Here's how the part is built. I have some questions about the finished solid (model axes, mm). A direction names the side the tool comes from. Round coordinates to 2 decimals unless told otherwise and drop trailing zeros. Order: outer loops, then holes, each group sorted by start corner. A loop starts at its lowest first (then second) coordinate and runs counter-clockwise, first axis right, second up.
```python
from build123d import *

# Parameters (mm, degrees)
SKETCH3_W           = 25.4
SKETCH3_H           = 25.4
BOSS_EXTRUDE1_DEPTH = 76.8
SKETCH4_R           = 2.6035
CUT_EXTRUDE1_DEPTH  = 79.872175068
CUT_EXTRUDE2_DEPTH  = 79.872175068
FILLET1_R           = 2.54
FILLET2_R           = 1.778


with BuildPart() as part:
    # Sketch3 → Boss-Extrude1 (new body)
    with BuildSketch(Plane.XY):
        Rectangle(SKETCH3_W, SKETCH3_H)
    extrude(amount=BOSS_EXTRUDE1_DEPTH)

    # Sketch4 → Cut-Extrude1 (cut, through all)
    with BuildSketch(Plane.XY.offset(76.8)):
        with BuildLine():
            Line((3.2512, 12.7), (-3.2512, 12.7))
            Line((-3.2512, 12.7), (-3.2512, 10.4902))
            Line((-3.2512, 10.4902), (-6.348478019, 10.4902))
            ThreePointArc((-6.348478019, 10.4902), (-7.335478831, 9.830707141), (-7.103895736, 8.666460301))
            Line((-7.103895736, 8.666460301), (-2.958635435, 4.5212))
            Line((-2.958635435, 4.5212), (2.958635435, 4.5212))
            Line((2.958635435, 4.5212), (7.103895736, 8.666460301))
            ThreePointArc((7.103895736, 8.666460301), (7.335478831, 9.830707141), (6.348478019, 10.4902))
            Line((6.348478019, 10.4902), (3.2512, 10.4902))
            Line((3.2512, 10.4902), (3.2512, 12.7))
        make_face()
        with BuildLine():
            Line((12.7, -3.2512), (12.7, 3.2512))
            Line((12.7, 3.2512), (10.4902, 3.2512))
            Line((10.4902, 3.2512), (10.4902, 6.348478019))
            ThreePointArc((10.4902, 6.348478019), (9.830707141, 7.335478831), (8.666460301, 7.103895736))
            Line((8.666460301, 7.103895736), (4.5212, 2.958635435))
            Line((4.5212, 2.958635435), (4.5212, -2.958635435))
            Line((4.5212, -2.958635435), (8.666460301, -7.103895736))
            ThreePointArc((8.666460301, -7.103895736), (9.830707141, -7.335478831), (10.4902, -6.348478019))
            Line((10.4902, -6.348478019), (10.4902, -3.2512))
            Line((10.4902, -3.2512), (12.7, -3.2512))
        make_face()
        with BuildLine():
            Line((-3.2512, -10.4902), (-3.2512, -12.7))
            Line((-3.2512, -12.7), (3.2512, -12.7))
            Line((3.2512, -12.7), (3.2512, -10.4902))
            Line((3.2512, -10.4902), (6.348478019, -10.4902))
            ThreePointArc((6.348478019, -10.4902), (7.335478831, -9.830707141), (7.103895736, -8.666460301))
            Line((7.103895736, -8.666460301), (2.958635435, -4.5212))
            Line((2.958635435, -4.5212), (-2.958635435, -4.5212))
            Line((-2.958635435, -4.5212), (-7.103895736, -8.666460301))
            ThreePointArc((-7.103895736, -8.666460301), (-7.335478831, -9.830707141), (-6.348478019, -10.4902))
            Line((-6.348478019, -10.4902), (-3.2512, -10.4902))
        make_face()
        with BuildLine():
            Line((-10.4902, 3.2512), (-12.7, 3.2512))
            Line((-12.7, 3.2512), (-12.7, -3.2512))
            Line((-12.7, -3.2512), (-10.4902, -3.2512))
            Line((-10.4902, -3.2512), (-10.4902, -6.348478019))
            ThreePointArc((-10.4902, -6.348478019), (-9.830707141, -7.335478831), (-8.666460301, -7.103895736))
            Line((-8.666460301, -7.103895736), (-4.5212, -2.958635435))
            Line((-4.5212, -2.958635435), (-4.5212, 2.958635435))
            Line((-4.5212, 2.958635435), (-8.666460301, 7.103895736))
            ThreePointArc((-8.666460301, 7.103895736), (-9.830707141, 7.335478831), (-10.4902, 6.348478019))
            Line((-10.4902, 6.348478019), (-10.4902, 3.2512))
        make_face()
        Circle(SKETCH4_R)
    extrude(amount=-CUT_EXTRUDE1_DEPTH, mode=Mode.SUBTRACT)

    # Sketch5 → Cut-Extrude2 (cut, through all)
    with BuildSketch(Plane.XY.offset(76.8)):
        with BuildLine():
            ThreePointArc((-11.5951, 3.2512), (-12.376382283, 3.574817717), (-12.7, 4.3561))
            Line((-12.7, 4.3561), (-12.7, 3.2512))
            Line((-12.7, 3.2512), (-11.5951, 3.2512))
        make_face()
        with BuildLine():
            ThreePointArc((-10.4902, 4.3561), (-10.813817717, 3.574817717), (-11.5951, 3.2512))
            Line((-11.5951, 3.2512), (-10.4902, 3.2512))
            Line((-10.4902, 3.2512), (-10.4902, 4.3561))
        make_face()
        with BuildLine():
            Line((-12.7, -3.2512), (-12.7, -4.3561))
            ThreePointArc((-12.7, -4.3561), (-12.376382283, -3.574817717), (-11.5951, -3.2512))
            Line((-11.5951, -3.2512), (-12.7, -3.2512))
        make_face()
        with BuildLine():
            Line((-10.4902, -3.2512), (-11.5951, -3.2512))
            ThreePointArc((-11.5951, -3.2512), (-10.813817717, -3.574817717), (-10.4902, -4.3561))
            Line((-10.4902, -4.3561), (-10.4902, -3.2512))
        make_face()
        with BuildLine():
            Line((-3.2512, -11.595100007), (-3.2512, -10.4902))
            Line((-3.2512, -10.4902), (-4.3561, -10.4902))
            ThreePointArc((-4.3561, -10.4902), (-3.574817715, -10.81381772), (-3.2512, -11.595100007))
        make_face()
        with BuildLine():
            Line((-3.2512, -12.7), (-3.2512, -11.595100007))
            ThreePointArc((-3.2512, -11.595100007), (-3.57481772, -12.376382285), (-4.3561, -12.7))
            Line((-4.3561, -12.7), (-3.2512, -12.7))
        make_face()
        with BuildLine():
            Line((3.2512, -10.4902), (3.2512, -11.5951))
            ThreePointArc((3.2512, -11.5951), (3.574817718, -10.813817717), (4.3561, -10.4902))
            Line((4.3561, -10.4902), (3.2512, -10.4902))
        make_face()
        with BuildLine():
            Line((3.2512, -12.7), (4.3561, -12.7))
            ThreePointArc((4.3561, -12.7), (3.574817717, -12.376382282), (3.2512, -11.5951))
            Line((3.2512, -11.5951), (3.2512, -12.7))
        make_face()
        with BuildLine():
            Line((11.5951, -3.2512), (10.4902, -3.2512))
            Line((10.4902, -3.2512), (10.4902, -4.3561))
            ThreePointArc((10.4902, -4.3561), (10.813817717, -3.574817717), (11.5951, -3.2512))
        make_face()
        with BuildLine():
            Line((12.7, -3.2512), (11.5951, -3.2512))
            ThreePointArc((11.5951, -3.2512), (12.376382283, -3.574817717), (12.7, -4.3561))
            Line((12.7, -4.3561), (12.7, -3.2512))
        make_face()
        with BuildLine():
            Line((10.4902, 3.2512), (11.5951, 3.2512))
            ThreePointArc((11.5951, 3.2512), (10.813817717, 3.574817717), (10.4902, 4.3561))
            Line((10.4902, 4.3561), (10.4902, 3.2512))
        make_face()
        with BuildLine():
            Line((12.7, 3.2512), (12.7, 4.3561))
            ThreePointArc((12.7, 4.3561), (12.376382283, 3.574817717), (11.5951, 3.2512))
            Line((11.5951, 3.2512), (12.7, 3.2512))
        make_face()
        with BuildLine():
            Line((3.2512, 12.7), (3.2512, 11.595099996))
            ThreePointArc((3.2512, 11.595099996), (3.574817716, 12.376382281), (4.3561, 12.7))
            Line((4.3561, 12.7), (3.2512, 12.7))
        make_face()
        with BuildLine():
            Line((3.2512, 11.595099996), (3.2512, 10.4902))
            Line((3.2512, 10.4902), (4.3561, 10.4902))
            ThreePointArc((4.3561, 10.4902), (3.574817719, 10.813817716), (3.2512, 11.595099996))
        make_face()
        with BuildLine():
            Line((-3.2512, 12.7), (-4.3561, 12.7))
            ThreePointArc((-4.3561, 12.7), (-3.574817717, 12.376382283), (-3.2512, 11.5951))
            Line((-3.2512, 11.5951), (-3.2512, 12.7))
        make_face()
        with BuildLine():
            Line((-3.2512, 10.4902), (-3.2512, 11.5951))
            ThreePointArc((-3.2512, 11.5951), (-3.574817717, 10.813817717), (-4.3561, 10.4902))
            Line((-4.3561, 10.4902), (-3.2512, 10.4902))
        make_face()
        with BuildLine():
            ThreePointArc((-12.7, 5.23875), (-12.14755, 5.7912), (-12.7, 6.34365))
            Line((-12.7, 6.34365), (-12.7, 5.23875))
        make_face()
        with BuildLine():
            ThreePointArc((-12.7, 9.60755), (-12.14755, 10.16), (-12.7, 10.71245))
            Line((-12.7, 10.71245), (-12.7, 9.60755))
        make_face()
        with BuildLine():
            ThreePointArc((-10.71245, 12.7), (-10.16, 12.14755), (-9.60755, 12.7))
            Line((-9.60755, 12.7), (-10.71245, 12.7))
        make_face()
        with BuildLine():
            ThreePointArc((-6.34365, 12.7), (-5.7912, 12.14755), (-5.23875, 12.7))
            Line((-5.23875, 12.7), (-6.34365, 12.7))
        make_face()
        with BuildLine():
            Line((6.34365, 12.7), (5.23875, 12.7))
            ThreePointArc((5.23875, 12.7), (5.7912, 12.14755), (6.34365, 12.7))
        make_face()
        with BuildLine():
            Line((10.71245, 12.7), (9.60755, 12.7))
            ThreePointArc((9.60755, 12.7), (10.16, 12.14755), (10.71245, 12.7))
        make_face()
        with BuildLine():
            Line((12.7, 10.71245), (12.7, 9.60755))
            ThreePointArc((12.7, 9.60755), (12.14755, 10.16), (12.7, 10.71245))
        make_face()
        with BuildLine():
            Line((12.7, 6.34365), (12.7, 5.23875))
            ThreePointArc((12.7, 5.23875), (12.14755, 5.7912), (12.7, 6.34365))
        make_face()
        with BuildLine():
            Line((-12.7, -6.34365), (-12.7, -5.23875))
            ThreePointArc((-12.7, -5.23875), (-12.14755, -5.7912), (-12.7, -6.34365))
        make_face()
        with BuildLine():
            Line((-12.7, -10.71245), (-12.7, -9.60755))
            ThreePointArc((-12.7, -9.60755), (-12.14755, -10.16), (-12.7, -10.71245))
        make_face()
        with BuildLine():
            Line((-10.71245, -12.7), (-9.60755, -12.7))
            ThreePointArc((-9.60755, -12.7), (-10.16, -12.14755), (-10.71245, -12.7))
        make_face()
        with BuildLine():
            Line((-6.34365, -12.7), (-5.23875, -12.7))
            ThreePointArc((-5.23875, -12.7), (-5.7912, -12.14755), (-6.34365, -12.7))
        make_face()
        with BuildLine():
            Line((12.7, -10.71245), (12.7, -9.60755))
            ThreePointArc((12.7, -9.60755), (12.14755, -10.16), (12.7, -10.71245))
        make_face()
        with BuildLine():
            Line((12.7, -6.34365), (12.7, -5.23875))
            ThreePointArc((12.7, -5.23875), (12.14755, -5.7912), (12.7, -6.34365))
        make_face()
        with BuildLine():
            Line((10.71245, -12.7), (9.60755, -12.7))
            ThreePointArc((9.60755, -12.7), (10.16, -12.14755), (10.71245, -12.7))
        make_face()
        with BuildLine():
            Line((6.34365, -12.7), (5.23875, -12.7))
            ThreePointArc((5.23875, -12.7), (5.7912, -12.14755), (6.34365, -12.7))
        make_face()
    extrude(amount=-CUT_EXTRUDE2_DEPTH, mode=Mode.SUBTRACT)

    # Fillet1
    fillet1_edges = [part.edges().sort_by_distance(p)[0] for p in [
        (-2.958635435, -4.5212, 38.4),
        (2.958635435, -4.5212, 38.4),
        (4.5212, -2.958635435, 38.4),
        (4.5212, 2.958635435, 38.4),
        (-4.5212, 2.958635435, 38.4),
        (-4.5212, -2.958635435, 38.4),
        (2.958635435, 4.5212, 38.4),
        (-2.958635435, 4.5212, 38.4),
    ]]
    fillet(fillet1_edges, radius=FILLET1_R)

    # Fillet2
    fillet2_edges = [part.edges().sort_by_distance(p)[0] for p in [
        (-12.7, 12.7, 38.4),
        (12.7, 12.7, 38.4),
        (12.7, -12.7, 38.4),
        (-12.7, -12.7, 38.4),
    ]]
    fillet(fillet2_edges, radius=FILLET2_R)


solid = part.part
```
1) We'd pull the mould along X, two halves only. Please class faces 1 (the cylindrical face through (9.847, 7.329, 38.938)), 2 (the flat face through (12.7, -8, 38)), 3 (the flat face through (-8, 12.7, 38)): +X half, -X half, draft (parallel to the pull), parting line (faces both ways), or undercut.
2) I need wall thicknesses on line 1 (Y direction, x = 0, z = 58); line 2 (Y direction, x = -3.5, z = 69); line 3 (X direction, y = 5, z = 24.5). Which ranges of each line are inside material? Lowest first, please.
3) I'm going to push flat-ended pins straight in: pin 1 (1.9 mm diameter, centred on x = -1, z = 22.5, fed in from +Y); pin 2 (3 mm diameter, centred on y = 0, z = 46, fed in from +X); pin 3 (4 mm diameter, centred on y = -1, z = 32.5, fed in from -X). Where does each tip first touch, or does it pass through?
4) For faces 4 (the flat face through (-4.521, 0, 39)), 5 (the flat face through (0, 3, 76.8)), 6 (the cylindrical face through (4.72, 2.89, 37.86)), which set-ups out of +Z, -Z, +X, -X, +Y, -Y let a thin tool reach every point of the face, with its end or its side?
5) If we section it at A-A (y = 0): Write out the boundary of the cut face in (x, z), plus the area to 3 significant figures.
Solutions:
1. face 1: undercut
1. face 2: +X half
1. face 3: draft
2. line 1: y = -4.52 to -2.6, 2.6 to 4.52
2. line 2: y = -12.29 to -10.9, -5.08 to 5.08, 10.9 to 12.29
2. line 3: x = -12.7 to -10.49, -6.56 to -3.39, 3.39 to 6.56, 10.49 to 12.7
3. pin 1: stops at y = 4.52
3. pin 2: stops at x = 4.52
3. pin 3: stops at x = -4.77
4. face 4: +Z, -Z, -X
4. face 5: +Z, +X, -X, +Y, -Y
4. face 6: +Z, -Z
5. outline: (-4.52, 0) - (-2.6, 0) - (-2.6, 76.8) - (-4.52, 76.8) - close; (2.6, 0) - (4.52, 0) - (4.52, 76.8) - (2.6, 76.8) - close
5. area: 295 mm2
